For this review, take the finished solid that the model builds, in its own axes (mm). Give positions to 0.01 mm unless a question says otherwise; leave off trailing zeros. Write each loop counter-clockwise with the first axis right and the second up, starting at its lowest first coordinate (ties: lowest second). Pieces come first, ordered by that corner, then holes.
Q1. We need section C-C (y = 56.5). Write out the cut boundary in (x, z).
Q2. We need section D-D (y = 22.5). Write out the cut boundary in (x, z), then the cut area to 4 significant figures.
Q3. We need section B-B (x = 50). Write out the cut boundary in (y, z), then the cut area to 3 significant figures.
Q4. We need section A-A (y = 90). Write out the cut boundary in (x, z), then the cut area to 3 significant figures.
Q5. Insertion check: P1, Ø4, axis at x = 62.5, y = 18.5, coming from the +Z side; P2, Ø1.8, axis at y = 73.5, z = 8, coming from the +X side; P3, Ø1, axis at x = 79, z = 3.5, coming from the +Y side; P4, Ø2, axis at x = 80, y = 13.2, coming from the -Z side. Each pin has a flat end and moves straight along its axis. Give the tip position at first contact, or say it passes through.
Q6. For line 1 (Y direction, x = 80, z = 6.15); line 2 (X direction, y = 53, z = 6); line 3 (Z direction, x = 23.5, y = 75.5), list the stretches that pass through material, from the lowest coordinate up.
```python
from build123d import *

# Parameters (mm, degrees)
PAD_DEPTH       = 8.6
SKETCH001_R     = 1.8
SKETCH001_R_2   = 1.73
POCKET_DEPTH    = 8.601
POCKET001_DEPTH = 1.6
POCKET002_DEPTH = 5
CHAMFER_SIZE    = 1


with BuildPart() as part:
    # Sketch → Pad (new body)
    with BuildSketch(Plane.XY):
        Polygon((0, 0), (0, 100), (25, 100), (25, 25), (100, 25), (100, 0), align=None)
    extrude(amount=PAD_DEPTH)

    # Sketch001 → Pocket (cut, through all)
    with BuildSketch(Plane.XY.offset(8.6)):
        with Locations((10, 10)):
            Circle(SKETCH001_R)
        with Locations((80, 13.2)):
            Circle(SKETCH001_R_2)
        with Locations((13.2, 80)):
            Circle(SKETCH001_R_2)
        with BuildLine():
            ThreePointArc((9.75, 51.8), (7.95, 50), (9.75, 48.2))
            Line((9.75, 48.2), (10.25, 48.2))
            ThreePointArc((10.25, 48.2), (12.05, 50), (10.25, 51.8))
            Line((9.75, 51.8), (10.25, 51.8))
        make_face()
        with BuildLine():
            ThreePointArc((9.5, 91.8), (7.7, 90), (9.5, 88.2))
            Line((9.5, 88.2), (10.5, 88.2))
            ThreePointArc((10.5, 88.2), (12.3, 90), (10.5, 91.8))
            Line((9.5, 91.8), (10.5, 91.8))
        make_face()
        with BuildLine():
            ThreePointArc((51.8, 10.25), (50, 12.05), (48.2, 10.25))
            Line((48.2, 10.25), (48.2, 9.75))
            ThreePointArc((48.2, 9.75), (50, 7.95), (51.8, 9.75))
            Line((51.8, 10.25), (51.8, 9.75))
        make_face()
        with BuildLine():
            ThreePointArc((91.8, 10.5), (90, 12.3), (88.2, 10.5))
            Line((88.2, 10.5), (88.2, 9.5))
            ThreePointArc((88.2, 9.5), (90, 7.7), (91.8, 9.5))
            Line((91.8, 10.5), (91.8, 9.5))
        make_face()
    extrude(amount=-POCKET_DEPTH, mode=Mode.SUBTRACT)

    # Sketch002 → Pocket001 (cut)
    with BuildSketch(Plane.XY.offset(8.6)):
        with BuildLine():
            Line((15, 110), (110, 110))
            Line((110, 110), (110, 15))
            Line((110, 15), (18.645751, 15))
            ThreePointArc((15, 18.645751), (14, 14), (18.645751, 15))
            Line((15, 18.645751), (15, 110))
        make_face()
    extrude(amount=-POCKET001_DEPTH, mode=Mode.SUBTRACT)

    # Sketch003 → Pocket002 (cut)
    with BuildSketch(Plane(origin=(0, 0, 0), x_dir=(1, 0, 0), z_dir=(0, 0, -1))):
        Polygon((81.80356, -15.813523), (83.165158, -12.944833), (81.361598, -10.331309), (78.19644, -10.586477), (76.834842, -13.455167), (78.638402, -16.068691), align=None)
        Polygon((16.374919, -80.056763), (14.836618, -77.278821), (11.661699, -77.222058), (10.025081, -79.943237), (11.563382, -82.721179), (14.738301, -82.777942), align=None)
    extrude(amount=-POCKET002_DEPTH, mode=Mode.SUBTRACT)

    # Chamfer
    chamfer_edges = [part.edges().sort_by_distance(p)[0] for p in [
        (50, 0, 8.6),
        (0, 50, 8.6),
        (50, 0, 0),
        (0, 0, 4.3),
        (100, 0, 4.3),
        (100, 7.5, 8.6),
        (100, 12.5, 0),
        (100, 25, 3.5),
        (25, 100, 3.5),
        (7.5, 100, 8.6),
        (0, 50, 0),
        (12.5, 100, 0),
        (25, 62.5, 0),
        (62.5, 25, 0),
        (0, 100, 4.3),
    ]]
    chamfer(chamfer_edges, length=CHAMFER_SIZE)


solid = part.part
```
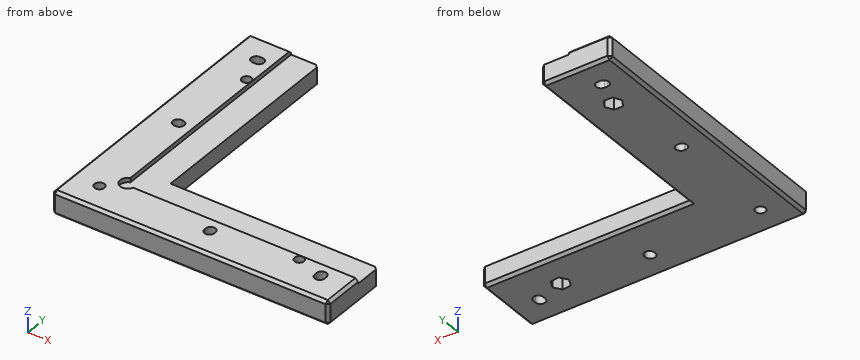
Computed:
1. outline: (0, 1) - (1, 0) - (24, 0) - (25, 1) - (25, 7) - (15, 7) - (15, 8.6) - (1, 8.6) - (0, 7.6) - close
2. outline: (0, 1) - (1, 0) - (99, 0) - (100, 1) - (100, 7) - (15, 7) - (15, 8.6) - (1, 8.6) - (0, 7.6) - close
2. area: 722.5 mm2
3. outline: (0, 1) - (1, 0) - (7.95, 0) - (7.95, 8.6) - (1, 8.6) - (0, 7.6) - close; (12.05, 0) - (24, 0) - (25, 1) - (25, 7) - (15, 7) - (15, 8.6) - (12.05, 8.6) - close
3. area: 162 mm2
4. outline: (0, 1) - (1, 0) - (7.7, 0) - (7.7, 8.6) - (1, 8.6) - (0, 7.6) - close; (12.3, 0) - (24, 0) - (25, 1) - (25, 7) - (15, 7) - (15, 8.6) - (12.3, 8.6) - close
4. area: 158 mm2
5. P1: stops at z = 7
5. P2: stops at x = 15
5. P3: stops at y = 25
5. P4: passes through
6. line 1: y = 0 to 11.47, 14.93 to 25
6. line 2: x = 0 to 25
6. line 3: z = 0 to 7
